```python
from build123d import *

# Parameters (mm, degrees)
F0_R     = 31.75
F1_DEPTH = 101.6
F2_R     = 31.75
F3_DEPTH = 25.4


with BuildPart() as f1:
    # F0 (on Front) → F1 (new body)
    with BuildSketch(Plane.XZ):
        with BuildLine():
            ThreePointArc((6.401351, 40.312523), (5.106646, 43.076548), (3.381897, 45.594749))
            ThreePointArc((3.381897, 45.594749), (2.604737, 45.645742), (1.826821, 45.683489))
            ThreePointArc((1.826821, 45.683489), (-0.173197, 43.377838), (-1.773928, 40.779038))
            Line((-1.773928, 40.779038), (-1.766209, 40.601602))
            Line((-1.766209, 40.601602), (-1.545433, 35.526402))
            ThreePointArc((-1.545433, 35.526402), (-4.939165, 35.215313), (-8.287532, 34.580781))
            Line((-8.287532, 34.580781), (-9.512858, 39.693606))
            ThreePointArc((-9.512858, 39.693606), (-11.766756, 41.75177), (-14.32389, 43.418252))
            ThreePointArc((-14.32389, 43.418252), (-15.061406, 43.167956), (-15.794552, 42.905134))
            ThreePointArc((-15.794552, 42.905134), (-16.759993, 40.009617), (-17.244358, 36.996066))
            Line((-17.244358, 36.996066), (-15.023159, 32.230704))
            ThreePointArc((-15.023159, 32.230704), (-18.03951, 30.64457), (-20.890174, 28.776974))
            Line((-20.890174, 28.776974), (-23.97882, 33.031697))
            ThreePointArc((-23.97882, 33.031697), (-26.848775, 34.070663), (-29.848994, 34.631719))
            ThreePointArc((-29.848994, 34.631719), (-30.434587, 34.118241), (-31.011347, 33.594862))
            ThreePointArc((-31.011347, 33.594862), (-30.795232, 30.550294), (-30.089491, 27.580778))
            Line((-30.089491, 27.580778), (-26.213746, 24.028174))
            ThreePointArc((-26.213746, 24.028174), (-28.393504, 21.408469), (-30.312475, 18.592134))
            Line((-30.312475, 18.592134), (-34.794224, 21.341012))
            ThreePointArc((-34.794224, 21.341012), (-37.843312, 21.202607), (-40.82986, 20.572821))
            ThreePointArc((-40.82986, 20.572821), (-41.174377, 19.874332), (-41.506946, 19.170076))
            ThreePointArc((-41.506946, 19.170076), (-40.142176, 16.439967), (-38.353772, 13.966567))
            Line((-38.353772, 13.966567), (-33.413527, 12.167572))
            ThreePointArc((-33.413527, 12.167572), (-34.424843, 8.913123), (-35.119977, 5.57681))
            Line((-35.119977, 5.57681), (-40.312523, 6.401351))
            ThreePointArc((-40.312523, 6.401351), (-43.076548, 5.106646), (-45.594749, 3.381897))
            ThreePointArc((-45.594749, 3.381897), (-45.645742, 2.604737), (-45.683489, 1.826821))
            ThreePointArc((-45.683489, 1.826821), (-43.377838, -0.173197), (-40.779038, -1.773928))
            Line((-40.779038, -1.773928), (-35.526402, -1.545433))
            ThreePointArc((-35.526402, -1.545433), (-35.215313, -4.939165), (-34.580781, -8.287532))
            Line((-34.580781, -8.287532), (-39.693606, -9.512858))
            ThreePointArc((-39.693606, -9.512858), (-41.75177, -11.766756), (-43.418252, -14.32389))
            ThreePointArc((-43.418252, -14.32389), (-43.167956, -15.061406), (-42.905134, -15.794552))
            ThreePointArc((-42.905134, -15.794552), (-40.009617, -16.759993), (-36.996066, -17.244358))
            Line((-36.996066, -17.244358), (-32.230704, -15.023159))
            ThreePointArc((-32.230704, -15.023159), (-30.64457, -18.03951), (-28.776974, -20.890174))
            Line((-28.776974, -20.890174), (-33.031697, -23.97882))
            ThreePointArc((-33.031697, -23.97882), (-34.070663, -26.848775), (-34.631719, -29.848994))
            ThreePointArc((-34.631719, -29.848994), (-34.118241, -30.434587), (-33.594862, -31.011347))
            ThreePointArc((-33.594862, -31.011347), (-30.550294, -30.795232), (-27.580778, -30.089491))
            Line((-27.580778, -30.089491), (-24.028174, -26.213746))
            ThreePointArc((-24.028174, -26.213746), (-21.408469, -28.393504), (-18.592134, -30.312475))
            Line((-18.592134, -30.312475), (-21.341012, -34.794224))
            ThreePointArc((-21.341012, -34.794224), (-21.202607, -37.843312), (-20.572821, -40.82986))
            ThreePointArc((-20.572821, -40.82986), (-19.874332, -41.174377), (-19.170076, -41.506946))
            ThreePointArc((-19.170076, -41.506946), (-16.439967, -40.142176), (-13.966567, -38.353772))
            Line((-13.966567, -38.353772), (-12.167572, -33.413527))
            ThreePointArc((-12.167572, -33.413527), (-8.913123, -34.424843), (-5.57681, -35.119977))
            Line((-5.57681, -35.119977), (-6.401351, -40.312523))
            ThreePointArc((-6.401351, -40.312523), (-5.106646, -43.076548), (-3.381897, -45.594749))
            ThreePointArc((-3.381897, -45.594749), (-2.604737, -45.645742), (-1.826821, -45.683489))
            ThreePointArc((-1.826821, -45.683489), (0.173197, -43.377838), (1.773928, -40.779038))
            Line((1.773928, -40.779038), (1.545433, -35.526402))
            ThreePointArc((1.545433, -35.526402), (4.939165, -35.215313), (8.287532, -34.580781))
            Line((8.287532, -34.580781), (9.512858, -39.693606))
            ThreePointArc((9.512858, -39.693606), (11.766756, -41.75177), (14.32389, -43.418252))
            ThreePointArc((14.32389, -43.418252), (15.061406, -43.167956), (15.794552, -42.905134))
            ThreePointArc((15.794552, -42.905134), (16.759993, -40.009617), (17.244358, -36.996066))
            Line((17.244358, -36.996066), (15.023159, -32.230704))
            ThreePointArc((15.023159, -32.230704), (18.03951, -30.64457), (20.890174, -28.776974))
            Line((20.890174, -28.776974), (23.97882, -33.031697))
            ThreePointArc((23.97882, -33.031697), (26.848775, -34.070663), (29.848994, -34.631719))
            ThreePointArc((29.848994, -34.631719), (30.434587, -34.118241), (31.011347, -33.594862))
            ThreePointArc((31.011347, -33.594862), (30.795232, -30.550294), (30.089491, -27.580778))
            Line((30.089491, -27.580778), (26.213746, -24.028174))
            ThreePointArc((26.213746, -24.028174), (28.393504, -21.408469), (30.312475, -18.592134))
            Line((30.312475, -18.592134), (34.794224, -21.341012))
            ThreePointArc((34.794224, -21.341012), (37.843312, -21.202607), (40.82986, -20.572821))
            ThreePointArc((40.82986, -20.572821), (41.174377, -19.874332), (41.506946, -19.170076))
            ThreePointArc((41.506946, -19.170076), (40.142176, -16.439967), (38.353772, -13.966567))
            Line((38.353772, -13.966567), (33.413527, -12.167572))
            ThreePointArc((33.413527, -12.167572), (34.424843, -8.913123), (35.119977, -5.57681))
            Line((35.119977, -5.57681), (40.312523, -6.401351))
            ThreePointArc((40.312523, -6.401351), (43.076548, -5.106646), (45.594749, -3.381897))
            ThreePointArc((45.594749, -3.381897), (45.645742, -2.604737), (45.683489, -1.826821))
            ThreePointArc((45.683489, -1.826821), (43.377838, 0.173197), (40.779038, 1.773928))
            Line((40.779038, 1.773928), (35.526402, 1.545433))
            ThreePointArc((35.526402, 1.545433), (35.215313, 4.939165), (34.580781, 8.287532))
            Line((34.580781, 8.287532), (39.693606, 9.512858))
            ThreePointArc((39.693606, 9.512858), (41.75177, 11.766756), (43.418252, 14.32389))
            ThreePointArc((43.418252, 14.32389), (43.167956, 15.061406), (42.905134, 15.794552))
            ThreePointArc((42.905134, 15.794552), (40.009617, 16.759993), (36.996066, 17.244358))
            Line((36.996066, 17.244358), (32.230704, 15.023159))
            ThreePointArc((32.230704, 15.023159), (30.64457, 18.03951), (28.776974, 20.890174))
            Line((28.776974, 20.890174), (33.031697, 23.97882))
            ThreePointArc((33.031697, 23.97882), (34.070663, 26.848775), (34.631719, 29.848994))
            ThreePointArc((34.631719, 29.848994), (34.118241, 30.434587), (33.594862, 31.011347))
            ThreePointArc((33.594862, 31.011347), (30.550294, 30.795232), (27.580778, 30.089491))
            Line((27.580778, 30.089491), (24.028174, 26.213746))
            ThreePointArc((24.028174, 26.213746), (21.408469, 28.393504), (18.592134, 30.312475))
            Line((18.592134, 30.312475), (21.341012, 34.794224))
            ThreePointArc((21.341012, 34.794224), (21.202607, 37.843312), (20.572821, 40.82986))
            ThreePointArc((20.572821, 40.82986), (19.874332, 41.174377), (19.170076, 41.506946))
            ThreePointArc((19.170076, 41.506946), (16.439967, 40.142176), (13.966567, 38.353772))
            Line((13.966567, 38.353772), (12.167572, 33.413527))
            ThreePointArc((12.167572, 33.413527), (8.913123, 34.424843), (5.57681, 35.119977))
            Line((5.57681, 35.119977), (6.373497, 40.137117))
            Line((6.373497, 40.137117), (6.401351, 40.312523))
        make_face()
        Circle(F0_R, mode=Mode.SUBTRACT)
        with BuildLine():
            ThreePointArc((6.471406, 40.121447), (6.436637, 40.21708), (6.401351, 40.312523))
            Line((6.401351, 40.312523), (6.373497, 40.137117))
            ThreePointArc((6.373497, 40.137117), (6.422456, 40.129312), (6.471406, 40.121447))
        make_face()
        with BuildLine():
            Line((-1.766209, 40.601602), (-1.773928, 40.779038))
            ThreePointArc((-1.773928, 40.779038), (-1.819842, 40.688229), (-1.865264, 40.597172))
            ThreePointArc((-1.865264, 40.597172), (-1.815738, 40.599417), (-1.766209, 40.601602))
        make_face()
    extrude(amount=F1_DEPTH)

    # F2 (on Front) → F3 (join)
    with BuildSketch(Plane.XZ):
        Circle(F2_R)
    extrude(amount=F3_DEPTH)


solid = f1.part
```
Design review of the part built by this model. Coordinates are the model's own, in mm. A direction names the side the tool comes from. Give positions to 0.01 mm unless a question says otherwise; leave off trailing zeros. Order: outer loops, then holes, each group sorted by start corner. A loop starts at its lowest first (then second) coordinate and runs counter-clockwise, first axis right, second up. Notation, with made-up numbers: (30, -1.5) -> (77, -1.5) arc R25 ccw to (77, 15.5) -> close; hole circle Ø10 at (15, 13). An arc over 180 degrees is marked (long way). Write each question's results on one line, items separated by ' | '. Start each with the question number.
Q1. For pin 1 (19 mm diameter, centred on x = 8, z = -3, fed in from -Y); pin 2 (8 mm diameter, centred on y = -55.5, z = -28, fed in from -X); pin 3 (1.5 mm diameter, centred on x = -20.5, y = -47.5, fed in from +Z), all flat-tipped, find the tip position at first contact; note any pin that passes through.
Q2. Add section B-B on x = 0. Give the boundary of the cut face in (y, z), and give its area (3 significant figures).
Q3. Wall thickness on L1, parallel to Z at x = 39, y = -96; L2, parallel to X at y = -45.5, z = -40.5; L3, parallel to Z at x = 0, y = -83: over which ranges is each line inside the solid? List them lowest first. Write a range as from..to.
Q4. Mouldability with a two-part tool opening along X and no side actions: class faces 1 (the cylindrical face through (34.06, -50.09, 26.81)), 2 (the flat face through (-25.83, -50.09, -28.18)), 3 (the flat face through (-17, -101.6, -27)), 4 (the flat face through (34.65, -50.09, 16.15)) as +X half, -X half, draft (parallel to the pull), parting line (faces both ways), or undercut.
Q5. Add section A-A on z = 0. Give the boundary of the cut face in (x, y).
Q6. Machinability: for faces 5 (the flat face through (37.68, -50.089, -5.983)), 6 (the flat face through (-13.08, -50.09, -35.92)), 7 (the cylindrical face through (-0.15, -50.09, 43.41)), which of the approach directions +Z, -Z, +X, -X, +Y, -Y give a long, thin tool a straight path to every point of the face, cutting with its end or side? Answer none if there is none.
Found:
1) pin 1: stops at y = -25.4 | pin 2: stops at x = -34.63 | pin 3: stops at z = 29.57
2) outline: (-101.6, -43.61) -> (0, -43.61) -> (0, 43.61) -> (-101.6, 43.61) -> (-101.6, 31.75) -> (-25.4, 31.75) -> (-25.4, -31.75) -> (-101.6, -31.75) -> close | area: 4,020 mm2
3) L1: z = -21.02..-14.77, -6.19..1.7, 9.35..16.98 | L2: x = -20.67..-17.06, -6.33..1.76, 10.31..16.63 | L3: z = -43.61..-31.75, 31.75..43.61
4) face 1: +X half | face 2: undercut | face 3: draft | face 4: undercut
5) outline: (-43.61, -101.6) -> (-31.75, -101.6) -> (-31.75, -25.4) -> (31.75, -25.4) -> (31.75, -101.6) -> (43.61, -101.6) -> (43.61, 0) -> (-43.61, 0) -> close
6) face 5: +Y, -Y | face 6: -Z, +Y, -Y | face 7: +Z, +Y, -Y
